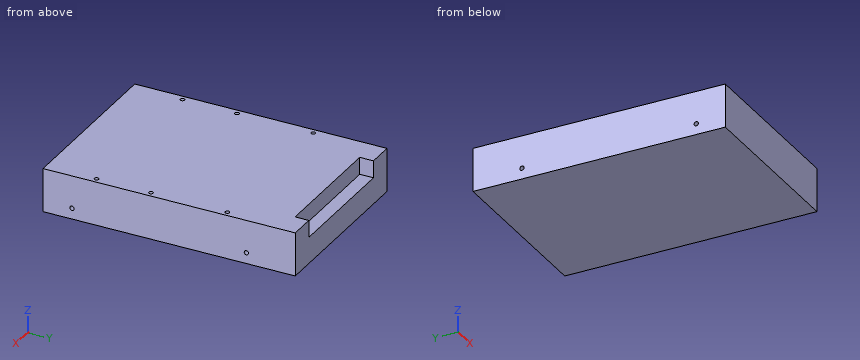
from build123d import *

# Parameters (mm, degrees)
F0_W     = 101.6
F0_H     = 147
F1_DEPTH = 25.4
F2_R     = 1.25
F2_W     = 71.6
F2_H     = 8
F3_DEPTH = 10
F4_R     = 1.25
F5_DEPTH = 10


# Not quite as in the source:
# - a pattern or mirror of a feature is missing from the dataset's text; its kind, count and spacing are read off the source's solid


with BuildPart() as f1:
    # F0 (on Top) → F1 (new body)
    with BuildSketch(Plane.XY):
        with Locations((50.8, 73.5)):
            Rectangle(F0_W, F0_H)
    extrude(amount=F1_DEPTH)

    # F2 (on face) → F3 (cut)
    with BuildSketch(Plane.XY.offset(25.4)):
        with Locations((3.18, 29.52)):
            Circle(F2_R)
        with Locations((3.18, 61.27)):
            Circle(F2_R)
        with Locations((3.18, 105.72)):
            Circle(F2_R)
        with Locations((98.42, 29.52)):
            Circle(F2_R)
        with Locations((98.42, 61.27)):
            Circle(F2_R)
        with Locations((98.42, 105.72)):
            Circle(F2_R)
        with Locations((50.8, 143)):
            Rectangle(F2_W, F2_H)
    extrude(amount=-F3_DEPTH, mode=Mode.SUBTRACT)

    # F4 (on face) → F5 (cut)
    with BuildSketch(Plane(origin=(0, 0, 0), x_dir=(0, -1, 0), z_dir=(-1, 0, 0))):
        with Locations((-118.5, 6.35)):
            Circle(F4_R)
        with Locations((-16.9, 6.35)):
            Circle(F4_R)
    f5 = extrude(amount=-F5_DEPTH, mode=Mode.SUBTRACT)

    # F5_copies: F5 across plane
    add(f5.mirror(Plane(origin=(50.8, 0, 0), x_dir=(0, 0, 1), z_dir=(1, 0, 0))), mode=Mode.SUBTRACT)


solid = f1.part
Check sheet for the modelled part. Datum: model origin and axes. Units: mm. Give positions to 0.01 mm unless a question says otherwise; leave off trailing zeros. Order: outer loops, then holes, each group sorted by start corner. A loop starts at its lowest first (then second) coordinate and runs counter-clockwise, first axis right, second up. Notation, with made-up numbers: M 70.25,-28.5 L 83.25,-28.5 A12 cw 83.25,-9.5 Z; hole C -19,3 d9. An arc over 180 degrees is marked long. Answer as CSV lines item,"result". Start each with the question number.
Item 1: Thickness scan on line 1 (Y direction, x = 3.18, z = 19.5); line 2 (X direction, y = 105.72, z = 17.5); line 3 (Y direction, x = 75, z = 20). Record the ranges inside material, lowest first. Write a range as [from, to].
Item 2: Gauge pin test, flat ends, axial feed: P1, Ø1.5, axis at x = 98.42, y = 29.52, coming from the +Z side; P2, Ø6, axis at x = 32.5, z = 13.5, coming from the -Y side; P3, Ø2, axis at y = 118.5, z = 6.35, coming from the -X side; P4, Ø2, axis at y = 16.9, z = 6.35, coming from the +X side. Record the tip position at first contact, or that the pin passes through.
Item 3: Cross-section at A-A on z = 19.5. Enter the section's corners in (x, y).
Item 4: Cross-section at B-B on x = 41. Enter the section's corners in (y, z).
Established:
1,line 1,"y = [0, 28.27], [30.77, 60.02], [62.52, 104.47], [106.97, 147]"
1,line 2,"x = [0, 1.93], [4.43, 97.17], [99.67, 101.6]"
1,line 3,"y = [0, 139]"
2,P1,"stops at z = 15.4"
2,P2,"stops at y = 0"
2,P3,"stops at x = 10"
2,P4,"stops at x = 91.6"
3,outline,"M 0,0 L 101.6,0 L 101.6,147 L 86.6,147 L 86.6,139 L 15,139 L 15,147 L 0,147 Z; hole C 3.18,29.52 d2.5; hole C 3.18,61.27 d2.5; hole C 3.18,105.72 d2.5; hole C 98.42,29.52 d2.5; hole C 98.42,61.27 d2.5; hole C 98.42,105.72 d2.5"
4,outline,"M 0,0 L 147,0 L 147,15.4 L 139,15.4 L 139,25.4 L 0,25.4 Z"
